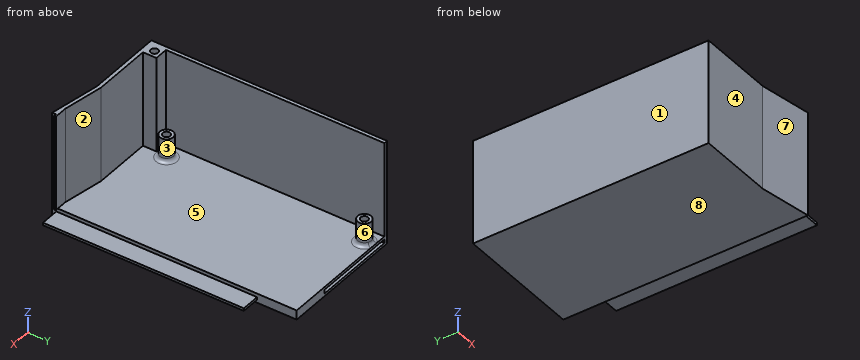
from build123d import *

# Parameters (mm, degrees)
SKETCH_1_W      = 63
SKETCH_1_H      = 116
PAD_DEPTH       = 5
PAD001_DEPTH    = 5
SKETCH001_W     = 5
SKETCH001_H     = 126.2
PAD002_DEPTH    = 5
PAD003_DEPTH    = 51
SKETCH003_W     = 7.2
SKETCH003_H     = 7.2
PAD004_DEPTH    = 51
SKETCH004_R     = 2
POCKET_DEPTH    = 6.7
SKETCH005_W     = 107.6
SKETCH005_H     = 1.4
PAD005_DEPTH    = 10
SKETCH006_R     = 3.6
PAD006_DEPTH    = 12.4
SKETCH007_R     = 2
POCKET001_DEPTH = 6.7
SKETCH008_W     = 45.1
SKETCH008_H     = 2.08
POCKET002_DEPTH = 11
PAD007_DEPTH    = 51
FILLET_R        = 2


with BuildPart() as part:
    # Sketch_1 → Pad (new body)
    with BuildSketch(Plane.XY):
        with Locations((-31.5, 58)):
            Rectangle(SKETCH_1_W, SKETCH_1_H)
    extrude(amount=PAD_DEPTH)

    # Sketch → Pad001 (join)
    with BuildSketch(Plane.XY):
        Polygon((0, 0), (-63, 0), (-63, -10.2), (-27.222153, -10.2), (0, -15), align=None)
    extrude(amount=PAD001_DEPTH)

    # Sketch001 → Pad002 (join)
    with BuildSketch(Plane.XY):
        with Locations((-65.5, 52.9)):
            Rectangle(SKETCH001_W, SKETCH001_H)
    extrude(amount=PAD002_DEPTH)

    # Sketch002 (on Face8 of Pad002) → Pad003 (join)
    with BuildSketch(Plane.XY.offset(5)):
        Polygon((-68, 116), (-68, -10.2), (-27.222153, -10.2), (0, -15), (0, -13), (-27.222153, -8.2), (-66, -8.2), (-66, 116), align=None)
    extrude(amount=PAD003_DEPTH)

    # Sketch003 (on Face8 of Pad003) → Pad004 (join)
    with BuildSketch(Plane.XY.offset(5)):
        with Locations((-62.4, -4.6)):
            Rectangle(SKETCH003_W, SKETCH003_H)
    extrude(amount=PAD004_DEPTH)

    # Sketch004 (on Face25 of Pad004) → Pocket (cut)
    with BuildSketch(Plane.XY.offset(56)):
        with Locations((-62.4, -4.6)):
            Circle(SKETCH004_R)
    extrude(amount=-POCKET_DEPTH, mode=Mode.SUBTRACT)

    # Sketch005 (on Face3 of Pocket) → Pad005 (join)
    with BuildSketch(Plane.YZ):
        with Locations((41, 2.36)):
            Rectangle(SKETCH005_W, SKETCH005_H)
    extrude(amount=PAD005_DEPTH)

    # Sketch006 (on Face5 of Pad005) → Pad006 (join)
    with BuildSketch(Plane.XY.offset(5)):
        with Locations((-58, 5)):
            Circle(SKETCH006_R)
        with Locations((-58, 111)):
            Circle(SKETCH006_R)
    extrude(amount=PAD006_DEPTH)

    # Sketch007 (on Face31 of Pad006) → Pocket001 (cut)
    with BuildSketch(Plane.XY.offset(17.4)):
        with Locations((-58, 5)):
            Circle(SKETCH007_R)
        with Locations((-58, 111)):
            Circle(SKETCH007_R)
    extrude(amount=-POCKET001_DEPTH, mode=Mode.SUBTRACT)

    # Sketch008 (on Face1 of Pocket001) → Pocket002 (cut)
    with BuildSketch(Plane(origin=(0, 116, 0), x_dir=(-1, 0, 0), z_dir=(0, 1, 0))):
        with Locations((43.5, 2.46)):
            Rectangle(SKETCH008_W, SKETCH008_H)
    extrude(amount=-POCKET002_DEPTH, mode=Mode.SUBTRACT)

    # Sketch009 (on Face15 of Pocket002) → Pad007 (join)
    with BuildSketch(Plane.XY.offset(5)):
        Polygon((0, -12), (-5.671282, -12), (0, -13), (1.5, -13), (1.5, -12), align=None)
    extrude(amount=PAD007_DEPTH)

    # Fillet
    fillet_edges = [part.edges().sort_by_distance(p)[0] for p in [
        (-61.6, 111, 5),
        (-61.6, 5, 5),
    ]]
    fillet(fillet_edges, radius=FILLET_R)


solid = part.part
Read the model definition and answer for the solid it produces. Units are mm, in the model's axes. Face numbers are marked on the shaded views. A direction names the side the tool comes from. Round coordinates to 2 decimals unless told otherwise and drop trailing zeros. Loops run counter-clockwise (first coordinate to the right, second up) from the corner with the lowest first, then second, coordinate; pieces in that order, holes last.
Q1. Section C-C on y = -4.6 is taken. Write down the section's boundary in (x, z), and give its area (3 significant figures).
Q2. Which of the six approach directions +Z, -Z, +X, -X, +Y, -Y give full straight-line access (tool end or side, diameter ignored) to the marked faces 1, 2, 3 and 4?
Q3. Each of these flat-tipped pins is pushed along its axis until it touches: pin 1 (9.5 mm diameter, centred on x = -40.5, z = 39, fed in from +Y); pin 2 (3.5 mm diameter, centred on y = -3.5, z = 38.5, fed in from +X); pin 3 (2 mm diameter, centred on x = -31, y = 70.5, fed in from +Z). Where does it stop, or does it pass through?
Q4. Consider probe 1 along Y at (x, z) = (-58, 15); probe 2 along Y at (x, z) = (-62.4, 51.75); probe 3 along Z at (x, y) = (-30.5, 108). Determine where each line is inside the solid, lowest interval first.
Q5. Section B-B on y = 111 is taken. Write down the section's boundary in (x, z).
Q6. Section D-D on y = 84.5 is taken. Write down the section's boundary in (x, z), and give its area (3 significant figures).
Q7. Section A-A on z = 27 is taken. Write down the section's boundary in (x, y).
Q8. Determine the mould class of the marked faces 5, 6, 7 and 8 for opening direction Y: released by +Y, released by -Y, zero draft, split by the parting line, or undercut.
Output:
1. outline: (-68, 0) - (0, 0) - (0, 1.66) - (10, 1.66) - (10, 3.06) - (0, 3.06) - (0, 5) - (-58.8, 5) - (-58.8, 56) - (-60.4, 56) - (-60.4, 49.3) - (-64.4, 49.3) - (-64.4, 56) - (-68, 56) - close
1. area: 796 mm2
2. face 1: +Z, -Z, -X, +Y, -Y
2. face 2: +Z, +X, +Y
2. face 3: +Z
2. face 4: +Z, -Z, -X, -Y
3. pin 1: stops at y = -8.2
3. pin 2: stops at x = -58.8
3. pin 3: stops at z = 5
4. probe 1: y = -10.2 to -8.2, 1.4 to 3, 7 to 8.6, 107.4 to 109, 113 to 114.6
4. probe 2: y = -10.2 to -6.6, -2.6 to -1
4. probe 3: z = 0 to 1.42, 3.5 to 5
5. outline: (-68, 0) - (0, 0) - (0, 5) - (-52.4, 5) arc R2 cw to (-54.4, 7) - (-54.4, 17.4) - (-56, 17.4) - (-56, 10.7) - (-60, 10.7) - (-60, 17.4) - (-61.6, 17.4) - (-61.6, 7) arc R2 cw to (-63.6, 5) - (-66, 5) - (-66, 56) - (-68, 56) - close; hole (-66.05, 1.42) - (-20.95, 1.42) - (-20.95, 3.5) - (-66.05, 3.5) - close
6. outline: (-68, 0) - (0, 0) - (0, 1.66) - (10, 1.66) - (10, 3.06) - (0, 3.06) - (0, 5) - (-66, 5) - (-66, 56) - (-68, 56) - close
6. area: 456 mm2
7. outline: (-68, -10.2) - (-27.22, -10.2) - (0, -15) - (0, -13) - (1.5, -13) - (1.5, -12) - (-5.67, -12) - (-27.22, -8.2) - (-58.8, -8.2) - (-58.8, -1) - (-66, -1) - (-66, 116) - (-68, 116) - close
8. face 5: undercut
8. face 6: undercut
8. face 7: released by -Y
8. face 8: zero draft
